The model under review builds one solid part; all positions refer to its coordinate system, in mm. A direction names the side the tool comes from. Give positions to 0.01 mm unless a question says otherwise; leave off trailing zeros. Loops run counter-clockwise (first coordinate to the right, second up) from the corner with the lowest first, then second, coordinate; pieces in that order, holes last. Notation, with made-up numbers: M 79,39.25 L 136,39.25 A21 cw 136,54.25 Z; hole C 18,37 d10. An arc over 180 degrees is marked long. Put each result on its own line as item: value. Start each with the question number.
from build123d import *

# Parameters (mm, degrees)
BOSS_EXTRUDE1_DEPTH = 16.82
BOSS_EXTRUDE2_DEPTH = 9.17
SKETCH3_R           = 2
BOSS_EXTRUDE3_DEPTH = 0.85
SKETCH4_R           = 1.47
BOSS_EXTRUDE4_DEPTH = 9.15
CUT_EXTRUDE1_DEPTH  = 9.15
SKETCH7_R           = 7.076677912
SKETCH7_R_2         = 2.5
CUT_EXTRUDE2_DEPTH  = 1.8
SKETCH8_R           = 2.5
CUT_EXTRUDE3_DEPTH  = 0.55
SKETCH9_W           = 14.3
SKETCH9_H           = 12.28
SKETCH9_W_2         = 10.3
SKETCH9_H_2         = 8.28
CUT_EXTRUDE4_DEPTH  = 7.57
FILLET1_R           = 1
CHAMFER2_SIZE       = 0.25
SKETCH10_R          = 0.35
CUT_EXTRUDE5_DEPTH  = 0.8
SKETCH11_R          = 0.35
CUT_EXTRUDE6_DEPTH  = 0.8
FILLET2_R           = 0.2
SKETCH12_R          = 0.825
CUT_EXTRUDE7_DEPTH  = 1
CUT_EXTRUDE8_DEPTH  = 1.25
SKETCH14_W          = 1.939968983
SKETCH14_H          = 2
CUT_EXTRUDE9_DEPTH  = 1.25
CHAMFER3_SIZE       = 0.3


with BuildPart() as part:
    # Sketch1 → Boss-Extrude1 (new body)
    with BuildSketch(Plane.XY):
        with BuildLine():
            Line((53.676749567, -74.893540286), (60.426749567, -74.893540286))
            ThreePointArc((60.426749567, -74.893540286), (63.051749567, -79.893540286), (60.426749567, -84.893540286))
            Line((60.426749567, -84.893540286), (53.676749567, -84.893540286))
            ThreePointArc((53.676749567, -84.893540286), (51.051749567, -79.893540286), (53.676749567, -74.893540286))
        make_face()
    extrude(amount=-BOSS_EXTRUDE1_DEPTH)

    # Sketch2 → Boss-Extrude2 (add)
    with BuildSketch(Plane.XY):
        with BuildLine():
            Line((63.001749567, -84.033540286), (63.001749567, -75.753540286))
            ThreePointArc((63.001749567, -75.753540286), (62.767434992, -75.187854862), (62.201749567, -74.953540286))
            Line((62.201749567, -74.953540286), (51.901749567, -74.953540286))
            ThreePointArc((51.901749567, -74.953540286), (51.336064142, -75.187854862), (51.101749567, -75.753540286))
            Line((51.101749567, -75.753540286), (51.101749567, -84.033540286))
            ThreePointArc((51.101749567, -84.033540286), (51.336064142, -84.599225711), (51.901749567, -84.833540286))
            Line((51.901749567, -84.833540286), (62.201749567, -84.833540286))
            ThreePointArc((62.201749567, -84.833540286), (62.767434992, -84.599225711), (63.001749567, -84.033540286))
        make_face()
    extrude(amount=BOSS_EXTRUDE2_DEPTH)

    # Sketch3 → Boss-Extrude3 (add)
    with BuildSketch(Plane.XY.offset(9.17)):
        with Locations((57.051749567, -79.893540286)):
            Circle(SKETCH3_R)
    extrude(amount=BOSS_EXTRUDE3_DEPTH)

    # Sketch4 → Boss-Extrude4 (add)
    with BuildSketch(Plane.XY.offset(10.02)):
        with Locations((57.051749567, -79.893540286)):
            Circle(SKETCH4_R)
    extrude(amount=BOSS_EXTRUDE4_DEPTH)

    # Sketch5 → Cut-Extrude1 (cut)
    with BuildSketch(Plane.XY.offset(19.17)):
        Polygon((57.051749567, -80.863540286), (58.479364881, -80.863540286), (58.479364881, -81.63553805), (55.371975477, -81.63553805), (55.371975477, -80.863540286), align=None)
    extrude(amount=-CUT_EXTRUDE1_DEPTH, mode=Mode.SUBTRACT)

    # Sketch7 → Cut-Extrude2 (cut)
    with BuildSketch(Plane(origin=(0, 0, -16.82), x_dir=(-1, 0, 0), z_dir=(0, 0, -1))):
        with Locations((-57.051749567, -79.893540286)):
            Circle(SKETCH7_R)
        with Locations((-57.051749567, -79.893540286)):
            Circle(SKETCH7_R_2, mode=Mode.SUBTRACT)
        Polygon((-60.551749567, -79.143540286), (-60.851749567, -79.143540286), (-60.851749567, -79.893540286), (-60.851749567, -80.643540286), (-60.551749567, -80.643540286), align=None, mode=Mode.SUBTRACT)
        Polygon((-53.251749567, -79.143540286), (-53.251749567, -79.893540286), (-53.251749567, -80.643540286), (-53.551749567, -80.643540286), (-53.551749567, -79.143540286), align=None, mode=Mode.SUBTRACT)
    extrude(amount=-CUT_EXTRUDE2_DEPTH, mode=Mode.SUBTRACT)

    # Sketch8 → Cut-Extrude3 (cut)
    with BuildSketch(Plane(origin=(0, 0, -16.82), x_dir=(-1, 0, 0), z_dir=(0, 0, -1))):
        with Locations((-57.051749567, -79.893540286)):
            Circle(SKETCH8_R)
    extrude(amount=-CUT_EXTRUDE3_DEPTH, mode=Mode.SUBTRACT)

    # Sketch9 → Cut-Extrude4 (cut)
    with BuildSketch(Plane.XY.offset(8.37)):
        with Locations((57.051749567, -79.893540286)):
            Rectangle(SKETCH9_W, SKETCH9_H)
        with Locations((57.051749567, -79.893540286)):
            Rectangle(SKETCH9_W_2, SKETCH9_H_2, mode=Mode.SUBTRACT)
    extrude(amount=-CUT_EXTRUDE4_DEPTH, mode=Mode.SUBTRACT)

    # Fillet1
    fillet1_edges = [part.edges().sort_by_distance(p)[0] for p in [
        (51.901749567, -75.753540286, 4.585),
        (51.901749567, -84.033540286, 4.585),
        (62.201749567, -84.033540286, 4.585),
        (62.201749567, -75.753540286, 4.585),
    ]]
    fillet(fillet1_edges, radius=FILLET1_R)

    # Chamfer2
    chamfer2_edges = [part.edges().sort_by_distance(p)[0] for p in [
        (60.701749567, -80.643540286, -16.82),
        (60.701749567, -79.143540286, -16.82),
        (53.401749567, -80.643540286, -16.82),
        (53.401749567, -79.143540286, -16.82),
    ]]
    chamfer(chamfer2_edges, length=CHAMFER2_SIZE)

    # Sketch10 → Cut-Extrude5 (cut)
    with BuildSketch(Plane(origin=(60.851749567, 0, 0), x_dir=(0, 0, -1), z_dir=(1, 0, 0))):
        with Locations((15.996548304, -79.893540286)):
            Circle(SKETCH10_R)
    extrude(amount=-CUT_EXTRUDE5_DEPTH, mode=Mode.SUBTRACT)

    # Sketch11 → Cut-Extrude6 (cut)
    with BuildSketch(Plane(origin=(53.551749567, 0, 0), x_dir=(0, 0, -1), z_dir=(1, 0, 0))):
        with Locations((15.996548304, -79.893540286)):
            Circle(SKETCH11_R)
    extrude(amount=-CUT_EXTRUDE6_DEPTH, mode=Mode.SUBTRACT)

    # Fillet2
    fillet2_edges = [part.edges().sort_by_distance(p)[0] for p in [
        (59.551749567, -79.893540286, -16.27),
    ]]
    fillet(fillet2_edges, radius=FILLET2_R)

    # Sketch12 → Cut-Extrude7 (cut)
    with BuildSketch(Plane(origin=(0, 0, -16.27), x_dir=(-1, 0, 0), z_dir=(0, 0, -1))):
        with Locations((-57.051749567, -79.893540286)):
            Circle(SKETCH12_R)
    extrude(amount=-CUT_EXTRUDE7_DEPTH, mode=Mode.SUBTRACT)

    # Sketch13 → Cut-Extrude8 (cut)
    with BuildSketch(Plane(origin=(0, 0, -15.02), x_dir=(-1, 0, 0), z_dir=(0, 0, -1))):
        with BuildLine():
            Line((-53.392555226, -73.943540286), (-60.710943907, -73.943540286))
            ThreePointArc((-60.710943907, -73.943540286), (-64.001749567, -79.893540286), (-60.710943907, -85.843540286))
            Line((-60.710943907, -85.843540286), (-53.392555226, -85.843540286))
            ThreePointArc((-53.392555226, -85.843540286), (-50.101749567, -79.893540286), (-53.392555226, -73.943540286))
        make_face()
        with BuildLine():
            Line((-53.692358654, -74.943540286), (-60.411140479, -74.943540286))
            ThreePointArc((-60.411140479, -74.943540286), (-63.001749567, -79.893540286), (-60.411140479, -84.843540286))
            Line((-60.411140479, -84.843540286), (-53.692358654, -84.843540286))
            ThreePointArc((-53.692358654, -84.843540286), (-51.101749567, -79.893540286), (-53.692358654, -74.943540286))
        make_face(mode=Mode.SUBTRACT)
    extrude(amount=-CUT_EXTRUDE8_DEPTH, mode=Mode.SUBTRACT)

    # Sketch14 → Cut-Extrude9 (cut)
    with BuildSketch(Plane(origin=(0, 0, -15.02), x_dir=(-1, 0, 0), z_dir=(0, 0, -1))):
        with Locations((-62.346150018, -79.893540286)):
            Rectangle(SKETCH14_W, SKETCH14_H)
        with Locations((-51.757349116, -79.893540286)):
            Rectangle(SKETCH14_W, SKETCH14_H)
    extrude(amount=-CUT_EXTRUDE9_DEPTH, mode=Mode.SUBTRACT)

    # Chamfer3
    chamfer3_edges = [part.edges().sort_by_distance(p)[0] for p in [
        (57.051749567, -78.423540286, 19.17),
    ]]
    chamfer(chamfer3_edges, length=CHAMFER3_SIZE)


solid = part.part
(1) Draft analysis for pull direction X (two halves, no side actions). For faces 4 (the flat face through (56, -80, -16.27)), 5 (the flat face through (57, -84.894, -7)), 6 (the cylindrical face through (52.202, -83.748, 4.532)), state which applies: +X half, -X half, draft (parallel to the pull), parting line (faces both ways), or undercut.
(2) For faces 1 (the cylindrical face through (57.099, -78.424, 14.383)), 2 (the flat face through (62, -84, 0)), 3 (the flat face through (57, -80, -15.27)), list the 3-axis set-ups (+Z, -Z, +X, -X, +Y, -Y) from which the entire face can be reached by the end or side of a thin tool; tool diameter is ignored.
(3) We need section B-B, the plane y = -83.5. Write out the cut boundary in (x, z).
(4) To check wall thickness, follow L1, parallel to Z at x = 60, y = -82; L2, parallel to X at y = -78.75, z = 1; L3, parallel to Y at x = 57, z = 2. State the ranges of each line that lie inside material, in increasing order. Write a range as [from, to].
(5) We need section D-D, the plane z = 14. Write out the cut boundary in (x, y).
(6) We need section C-C, the plane x = 52.25. Write out the cut boundary in (y, z), plus the area to 3 significant figures.
(7) We need section A-A, the plane z = 2.5. Write out the cut boundary in (x, y), plus the area to 3 significant figures.
(8) Insertion check: pin 1 (4 mm diameter, centred on x = 57.5, z = 12.5, fed in from -Y); pin 2 (1 mm diameter, centred on x = 56.5, z = -14.5, fed in from +Y); pin 3 (1.8 mm diameter, centred on x = 57.5, y = -80, fed in from -Z); pin 4 (5 mm diameter, centred on x = 60, y = -79, fed in from +Z). Each pin has a flat end and moves straight along its axis. Give the tip position at first contact, or say it passes through.
Check sheet entries:
1. face 4: undercut
1. face 5: draft
1. face 6: -X half
2. face 1: +Z
2. face 2: -Z, +X, -Y
2. face 3: -Z
3. outline: M 51.1,0 L 52.24,0 L 52.24,-13.77 L 52.3,-13.77 L 52.3,-15.02 L 61.8,-15.02 L 61.8,-13.77 L 61.87,-13.77 L 61.87,0 L 63,0 L 63,0.8 L 62.09,0.8 L 62.09,8.37 L 63,8.37 L 63,9.17 L 51.1,9.17 L 51.1,8.37 L 52.02,8.37 L 52.02,0.8 L 51.1,0.8 Z
4. L1: z = [-15.02, 9.17]
4. L2: x = [51.9, 62.2]
4. L3: y = [-84.03, -75.75]
5. outline: M 55.95,-80.86 L 58.16,-80.86 A1.47 ccw long Z
6. outline: M -84.83,0 L -83.52,0 L -83.52,-13.77 L -83.43,-13.77 L -83.43,-15.02 L -80.89,-15.02 L -80.89,-13.77 L -78.89,-13.77 L -78.89,-15.02 L -76.36,-15.02 L -76.36,-13.77 L -76.27,-13.77 L -76.27,0 L -74.95,0 L -74.95,0.8 L -76,0.8 L -76,8.37 L -74.95,8.37 L -74.95,9.17 L -84.83,9.17 L -84.83,8.37 L -83.79,8.37 L -83.79,0.8 L -84.83,0.8 Z
6. area: 181 mm²
7. outline: M 51.9,-83.03 A1 ccw 52.9,-84.03 L 61.2,-84.03 A1 ccw 62.2,-83.03 L 62.2,-76.75 A1 ccw 61.2,-75.75 L 52.9,-75.75 A1 ccw 51.9,-76.75 Z
7. area: 84.4 mm²
8. pin 1: stops at y = -80.86
8. pin 2: stops at y = -74.94
8. pin 3: stops at z = -16.27
8. pin 4: stops at z = 19.17
